Here's how the part is built. I have some questions about the finished solid (model axes, mm). Face numbers are marked on the shaded views. A direction names the side the tool comes from. Round coordinates to 2 decimals unless told otherwise and drop trailing zeros. Write each loop counter-clockwise with the first axis right and the second up, starting at its lowest first coordinate (ties: lowest second). Pieces come first, ordered by that corner, then holes. Notation, with made-up numbers: (0.5, 24.5) -> (6.5, 24.5) arc R16 ccw to (6.5, 29.5) -> close; hole circle Ø9 at (19, 85). An arc over 180 degrees is marked (long way). Answer in a Markdown table with one row per item.
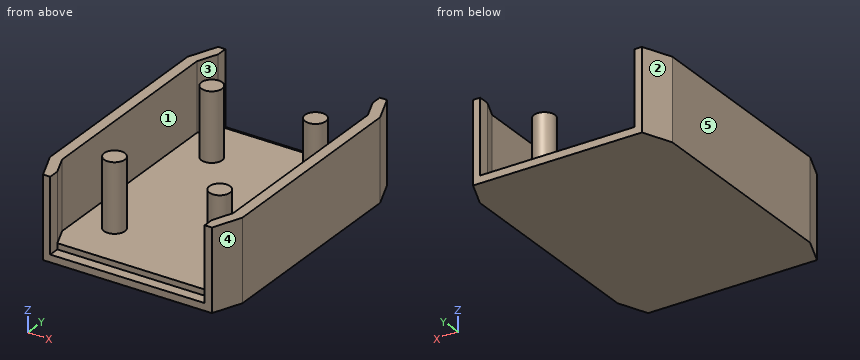
from build123d import *

# Parameters (mm, degrees)
BOSS_EXTRUDE1_DEPTH = 5.715
BOSS_EXTRUDE2_DEPTH = 29.21
SKETCH3_W           = 66.200858932
SKETCH3_H           = 4.6355
CUT_EXTRUDE1_DEPTH  = 31.75
SKETCH4_R           = 4.445
BOSS_EXTRUDE3_DEPTH = 29.21


with BuildPart() as part:
    # Sketch1 → Boss-Extrude1 (new body)
    with BuildSketch(Plane.XY):
        Polygon((41.275, 44.914422768), (36.195, 57.15), (-36.195, 57.15), (-41.275, 44.914422768), (-41.275, -44.914422768), (-36.195, -57.15), (36.195, -57.15), (41.275, -44.914422768), align=None)
    extrude(amount=BOSS_EXTRUDE1_DEPTH)

    # Sketch2 → Boss-Extrude2 (add)
    with BuildSketch(Plane.XY.offset(5.715)):
        Polygon((-41.275, 44.914422768), (-41.275, -44.914422768), (-36.195, -57.15), (36.195, -57.15), (41.275, -44.914422768), (41.275, 44.914422768), (36.195, 57.15), (-36.195, 57.15), align=None)
        Polygon((-33.100429466, 52.5145), (-36.6395, 43.99037188), (-36.6395, -43.99037188), (-33.100429466, -52.5145), (33.100429466, -52.5145), (36.6395, -43.99037188), (36.6395, 43.99037188), (33.100429466, 52.5145), align=None, mode=Mode.SUBTRACT)
    extrude(amount=BOSS_EXTRUDE2_DEPTH)

    # Sketch3 → Cut-Extrude1 (cut)
    with BuildSketch(Plane.XY.offset(34.925)):
        with Locations((0, 54.83225)):
            Rectangle(SKETCH3_W, SKETCH3_H)
    cut_extrude1 = extrude(amount=-CUT_EXTRUDE1_DEPTH, mode=Mode.SUBTRACT)

    # Mirror1: Cut-Extrude1 across plane
    add(cut_extrude1.mirror(Plane.ZX), mode=Mode.SUBTRACT)

    # Sketch4 → Boss-Extrude3 (add)
    with BuildSketch(Plane.XY.offset(5.715)):
        with Locations((22.874903427, -31.75)):
            Circle(SKETCH4_R)
        with Locations((-22.225, -31.75)):
            Circle(SKETCH4_R)
        with Locations((22.225, 31.75)):
            Circle(SKETCH4_R)
        with Locations((-22.225, 31.75)):
            Circle(SKETCH4_R)
    extrude(amount=BOSS_EXTRUDE3_DEPTH)


solid = part.part
1) I want a section at B-B, the plane y = 31.75. List the corners of the cut face in (x, z) for me (1 decimal), and give its area (3 significant figures).
Response:
| item | result |
|---|---|
| outline | (-41.3, 0) -> (41.3, 0) -> (41.3, 34.9) -> (36.6, 34.9) -> (36.6, 5.7) -> (26.7, 5.7) -> (26.7, 34.9) -> (17.8, 34.9) -> (17.8, 5.7) -> (-17.8, 5.7) -> (-17.8, 34.9) -> (-26.7, 34.9) -> (-26.7, 5.7) -> (-36.6, 5.7) -> (-36.6, 34.9) -> (-41.3, 34.9) -> close |
| area | 1,260 mm^2 |
2) Which directions (+Z, -Z, +X, -X, +Y, -Y) give clear straight access to the entire face, cutting with the end or side of a thin tool? Please do the marked faces 1 and 2.
Response:
| item | result |
|---|---|
| face 1 | +Z |
| face 2 | +Z, -Z, -X, +Y |
3) We'd pull the mould along Y, two halves only. Please class the marked faces 3, 4 and 5: +Y half, -Y half, draft (parallel to the pull), parting line (faces both ways), or undercut.
Response:
| item | result |
|---|---|
| face 3 | undercut |
| face 4 | -Y half |
| face 5 | draft |
4) For pin 1 (1.3 mm diameter, centred on x = -8.5, z = 5, fed in from +Y); pin 2 (5 mm diameter, centred on y = -55, z = 22, fed in from -X); pin 3 (1.4 mm diameter, centred on x = 10, y = 54.5, fed in from +Z) (3 decimals), each with a flat end and sliding along its axis, tell me the tip position at first contact or that it passes through.
Response:
| item | result |
|---|---|
| pin 1 | stops at y = 52.51 |
| pin 2 | stops at x = -38.13 |
| pin 3 | stops at z = 3.175 |
5) I need wall thicknesses on line 1 (X direction, y = -4.5, z = 29.5) (1 decimal); line 2 (X direction, y = 28.5, z = 23.5) (1 decimal); line 3 (Z direction, x = -30, y = 30) (3 decimals). Which ranges of each line are inside material? Lowest first, please. Write a range as [from, to].
Response:
| item | result |
|---|---|
| line 1 | x = [-41.3, -36.6], [36.6, 41.3] |
| line 2 | x = [-41.3, -36.6], [-25.3, -19.2], [19.2, 25.3], [36.6, 41.3] |
| line 3 | z = [0, 5.715] |
6) I want a section at D-D, the plane y = 19. List the corners of the cut face in (x, z) for me (1 decimal), and give its area (3 significant figures).
Response:
| item | result |
|---|---|
| outline | (-41.3, 0) -> (41.3, 0) -> (41.3, 34.9) -> (36.6, 34.9) -> (36.6, 5.7) -> (-36.6, 5.7) -> (-36.6, 34.9) -> (-41.3, 34.9) -> close |
| area | 743 mm^2 |
7) I want a section at A-A, the plane z = 15. Count the separate pieces of the cut face and the enclosed holes in it, and give its area (3 significant figures).
Response:
| item | result |
|---|---|
| separate pieces | 6 |
| enclosed holes | 0 |
| area | 1,310 mm^2 |
